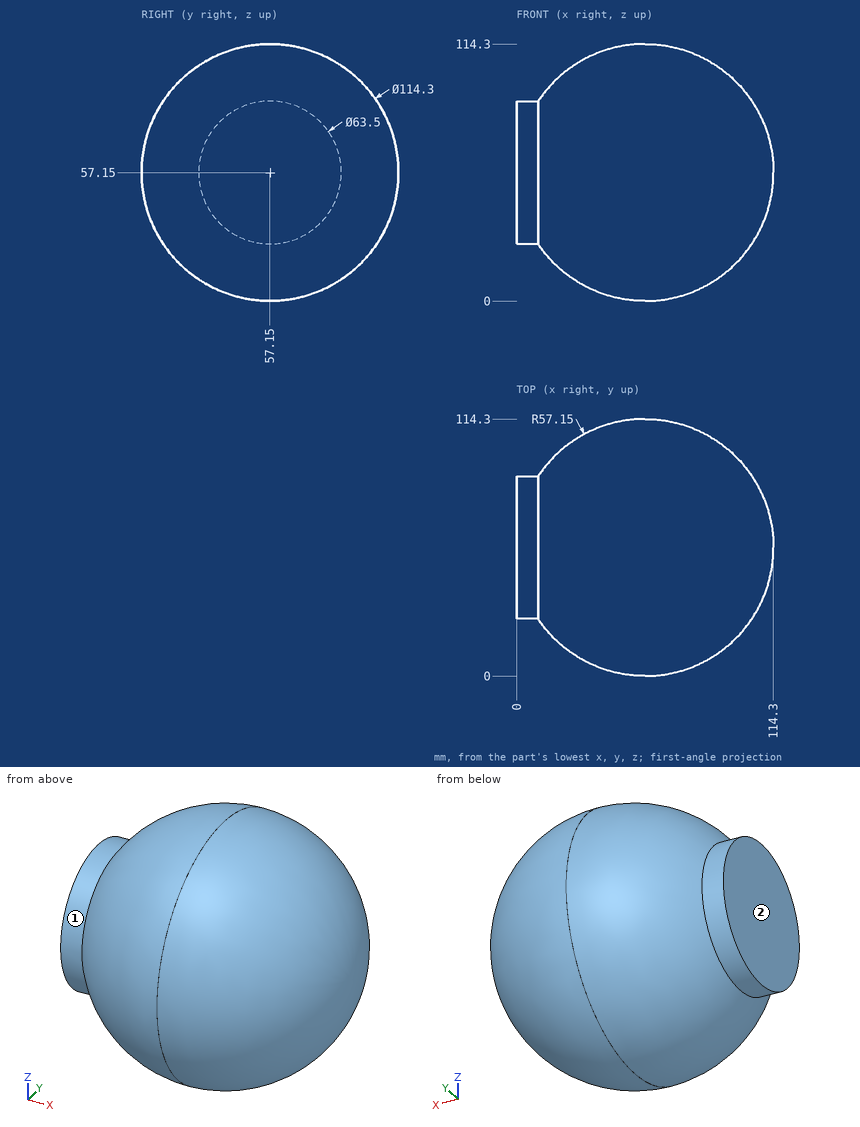
Study the drawing (mm; zero at the part's minimum x, y, z) and answer. A direction names the side the tool comes from. Round coordinates to 2 decimals unless told otherwise and drop trailing zeros. Use one line per item in the form item = value. Start each with the question number.
(1) Find the intervals of material crossed by line 1 along Z through (x, y) = (45, 97), in increasing order. Write a range as from..to.
(2) Flat-ended cylindrical pins translate along their axes: pin 1 Ø10 at (y, z) = (83.5, 79) entering from +X; pin 2 Ø5 at (x, y) = (30, 64.5) entering from -Z; pin 3 Ø8 at (x, z) = (92.5, 92) entering from +Y. Find the tip coordinate at first contact, or state that the pin passes through.
(3) For the marked faces 1 and 2, determine the directions among +Z, -Z, +X, -X, +Y, -Y from which every point of the face is accessible in a straight line to the end or side of a thin tool.
Checked values:
q1.line_1 = 18.03..96.27
q2.pin_1 = 106.26
q2.pin_2 = 6.07
q2.pin_3 = 91.55
q3.face_1 = -X
q3.face_2 = +Z, -Z, -X, +Y, -Y
